```python
from build123d import *

# Parameters (mm, degrees)
SKETCH1_W                = 12.7
SKETCH1_H                = 9.525
BOSS_EXTRUDE1_DEPTH      = 9.525
BOSS_EXTRUDE1_DEPTH_BACK = 22.225
SKETCH2_W                = 28.575
SKETCH2_H                = 32.144829198
CUT_EXTRUDE1_DEPTH       = 127.92060018
CUT_EXTRUDE1_DEPTH_BACK  = 127.92060018
CHAMFER1_SIZE            = 9.525
SKETCH11_W               = 143.179068554
SKETCH11_H               = 12.488767135
CUT_EXTRUDE5_DEPTH       = 119.773497618
SKETCH5_W                = 9.85
SKETCH5_H                = 3
SKETCH5_W_2              = 60
SKETCH5_H_2              = 4
CUT_EXTRUDE3_REACH       = 156.535
SKETCH6_R                = 1.7272
SKETCH6_R_2              = 8
SKETCH7_W                = 25.4
SKETCH7_H                = 22.769743879
BOSS_EXTRUDE2_DEPTH      = 1.5875
CUT_EXTRUDE4_REACH       = 157.713
SKETCH8_R                = 3
CUT_EXTRUDE6_DEPTH       = 99.74454178
CUT_EXTRUDE6_DEPTH_BACK  = 12.7


with BuildPart() as part:
    # Sketch1 → Revolve1 (revolve)
    with BuildSketch(Plane.XY, mode=Mode.PRIVATE) as revolve1_sk:
        with Locations((-28.575, 4.7625)):
            Rectangle(SKETCH1_W, SKETCH1_H)
        with Locations((28.575, 4.7625)):
            Rectangle(SKETCH1_W, SKETCH1_H)
    revolve(revolve1_sk.sketch.rotate(Axis((-22.225, 0, 0), (1, 0, 0)), 90), axis=Axis((-22.225, 0, 0), (1, 0, 0)))

    # Sketch2 → Boss-Extrude1 (add, two sides: drawn at the far end of the back side and taken through both)
    with BuildSketch(Plane(origin=(0, 0, 0), x_dir=(1, 0, 0), z_dir=(0, 1, 0)).offset(-BOSS_EXTRUDE1_DEPTH_BACK)):
        Polygon((-57.15, 5.955170802), (-34.925, 0), (-22.225, 0), (-22.225, 25.4), (22.225, 25.4), (22.225, 0), (34.925, 0), (57.15, 5.955170802), (57.15, 101.6), (-57.15, 101.6), align=None)
        Polygon((-22.225, 28.575), (-22.225, 50.8), (-53.975, 50.8), (-53.975, 98.425), (53.975, 98.425), (53.975, 50.8), (22.225, 50.8), (22.225, 28.575), align=None, mode=Mode.SUBTRACT)
        with Locations((39.6875, 28.377585401)):
            Rectangle(SKETCH2_W, SKETCH2_H, mode=Mode.SUBTRACT)
        with Locations((-39.6875, 28.377585401)):
            Rectangle(SKETCH2_W, SKETCH2_H, mode=Mode.SUBTRACT)
    extrude(amount=BOSS_EXTRUDE1_DEPTH + BOSS_EXTRUDE1_DEPTH_BACK)

    # Sketch3 → Cut-Extrude1 (cut, two sides: drawn at the far end of the back side and taken through both)
    with BuildSketch(Plane(origin=(0, 0, -101.6), x_dir=(-1, 0, 0), z_dir=(0, 0, -1)).offset(-CUT_EXTRUDE1_DEPTH_BACK)):
        Polygon((-363.181758486, 0.544743879), (-78.360804047, 0.544743879), (-53.975, 0.544743879), (-34.925, 9.525), (34.925, 9.525), (53.975, 0.544743879), (73.137213101, 0.544743879), (357.958167541, 0.544743879), (357.958167541, 570.186652758), (-363.181758486, 570.186652758), align=None)
    extrude(amount=CUT_EXTRUDE1_DEPTH + CUT_EXTRUDE1_DEPTH_BACK, mode=Mode.SUBTRACT)

    # Chamfer1
    chamfer1_edges = [part.edges().sort_by_distance(p)[0] for p in [
        (-25.4, -6.35, -12.305170802),
        (25.4, -6.35, -12.305170802),
    ]]
    chamfer(chamfer1_edges, length=CHAMFER1_SIZE)

    # Sketch11 → Cut-Extrude5 (cut, through all)
    with BuildSketch(Plane(origin=(0, 0.544743879, 0), x_dir=(1, 0, 0), z_dir=(0, 1, 0))):
        with Locations((14.439534277, 95.355616432)):
            Rectangle(SKETCH11_W, SKETCH11_H)
    extrude(amount=CUT_EXTRUDE5_DEPTH, mode=Mode.SUBTRACT)

    # Sketch5 → Cut-Revolve1 (revolve, cut)
    with BuildSketch(Plane(origin=(0, 0, 0), x_dir=(1, 0, 0), z_dir=(0, 1, 0)), mode=Mode.PRIVATE) as cut_revolve1_sk:
        Polygon((-34.925, -3), (-34.925, 0), (-41.275, 0), (-41.275, -6.604), (-34.925, -6.604), align=None)
        with Locations((-30, -1.5)):
            Rectangle(SKETCH5_W, SKETCH5_H)
        Polygon((73.349668225, 0), (34.925, 0), (34.925, -4), (34.925, -6.604), (73.349668225, -6.604), align=None)
        with Locations((4.925, -2)):
            Rectangle(SKETCH5_W_2, SKETCH5_H_2)
    revolve(cut_revolve1_sk.sketch.rotate(Axis((116.428907087, 0, 0), (-1, 0, 0)), 180), axis=Axis((116.428907087, 0, 0), (-1, 0, 0)), mode=Mode.SUBTRACT)

    # Sketch6 → Cut-Extrude3 (cut, up to next)
    with BuildSketch(Plane.ZY.offset(57.15), mode=Mode.PRIVATE) as cut_extrude3_sk1:
        with Locations((-88.9, -9.525)):
            Circle(SKETCH6_R)
    cut_extrude3_tool1 = extrude(cut_extrude3_sk1.sketch, amount=-CUT_EXTRUDE3_REACH, mode=Mode.PRIVATE) & part.part
    # Sketch6 → Cut-Extrude3 (cut, up to next)
    with BuildSketch(Plane.ZY.offset(57.15), mode=Mode.PRIVATE) as cut_extrude3_sk2:
        with Locations((-21.830170802, -9.525)):
            Circle(SKETCH6_R)
    cut_extrude3_tool2 = extrude(cut_extrude3_sk2.sketch, amount=-CUT_EXTRUDE3_REACH, mode=Mode.PRIVATE) & part.part
    # Sketch6 → Cut-Extrude3 (cut, up to next)
    with BuildSketch(Plane.ZY.offset(57.15), mode=Mode.PRIVATE) as cut_extrude3_sk3:
        with Locations((-55.365085401, -9.525)):
            Circle(SKETCH6_R_2)
    cut_extrude3_tool3 = extrude(cut_extrude3_sk3.sketch, amount=-CUT_EXTRUDE3_REACH, mode=Mode.PRIVATE) & part.part
    cut_extrude3_1 = cut_extrude3_tool1.solids().sort_by_distance((-57.15, -9.525, -88.9))[0]
    add(cut_extrude3_1, mode=Mode.SUBTRACT)
    cut_extrude3_2 = cut_extrude3_tool2.solids().sort_by_distance((-57.15, -9.525, -21.830171))[0]
    add(cut_extrude3_2, mode=Mode.SUBTRACT)
    cut_extrude3_3 = cut_extrude3_tool3.solids().sort_by_distance((-57.15, -9.525, -55.365085))[0]
    add(cut_extrude3_3, mode=Mode.SUBTRACT)
    cut_extrude3 = cut_extrude3_1 + cut_extrude3_2 + cut_extrude3_3  # Cut-Extrude3 as one shape, for the pattern or mirror that repeats it

    # Sketch7 → Boss-Extrude2 (add)
    with BuildSketch(Plane.ZY.offset(57.15)):
        with Locations((-55.365085401, -10.840128061)):
            Rectangle(SKETCH7_W, SKETCH7_H)
    boss_extrude2 = extrude(amount=BOSS_EXTRUDE2_DEPTH)

    # Sketch8 → Cut-Extrude4 (cut, up to next)
    with BuildSketch(Plane.ZY.offset(58.7375), mode=Mode.PRIVATE) as cut_extrude4_sk1:
        with Locations((-55.365085401, -9.525)):
            Circle(SKETCH8_R)
    cut_extrude4_tool1 = extrude(cut_extrude4_sk1.sketch, amount=-CUT_EXTRUDE4_REACH, mode=Mode.PRIVATE) & part.part
    cut_extrude4 = cut_extrude4_tool1.solids().sort_by_distance((-58.7375, -9.525, -55.365085))[0]
    add(cut_extrude4, mode=Mode.SUBTRACT)

    # Mirror1: Cut-Extrude3, Boss-Extrude2, Cut-Extrude4 across plane
    add(cut_extrude3.mirror(Plane(origin=(0, 0, 0), x_dir=(0, 0, 1), z_dir=(1, 0, 0))), mode=Mode.SUBTRACT)
    add(boss_extrude2.mirror(Plane(origin=(0, 0, 0), x_dir=(0, 0, 1), z_dir=(1, 0, 0))))
    add(cut_extrude4.mirror(Plane(origin=(0, 0, 0), x_dir=(0, 0, 1), z_dir=(1, 0, 0))), mode=Mode.SUBTRACT)

    # Sketch12 → Cut-Extrude6 (cut, two sides: drawn at the far end of the back side and taken through both)
    with BuildSketch(Plane.XY.offset(-25.4).offset(-CUT_EXTRUDE6_DEPTH_BACK)):
        Polygon((-139.974688472, 150.824626166), (-22.225, 9.525), (-6.35, -9.525), (6.35, -9.525), (22.225, 9.525), (139.974688472, 150.824626166), (139.974688472, 518.686412656), (-139.974688472, 518.686412656), align=None)
    extrude(amount=CUT_EXTRUDE6_DEPTH + CUT_EXTRUDE6_DEPTH_BACK, mode=Mode.SUBTRACT)


solid = part.part
```
CAD build for the part. Positions are in the model's coordinates, mm. A direction names the side the tool comes from. Round coordinates to 2 decimals unless told otherwise and drop trailing zeros. Loops run counter-clockwise (first coordinate to the right, second up) from the corner with the lowest first, then second, coordinate; pieces in that order, holes last. Notation, with made-up numbers: (4.25, 0.25) - (41.25, 0.25) arc R15 cw to (41.25, 10.25) - close; hole circle Ø8 at (-33, 12.25). An arc over 180 degrees is marked (long way). Return JSON: item names as keys, results as strings. Group by question number.
Q1. Flat gauge pins, fed straight in: pin 1 Ø16 at (y, z) = (-13, -11.5) entering from +X; pin 2 Ø1.3 at (x, y) = (-57.5, -10) entering from +Z; pin 3 Ø10 at (x, y) = (-10.5, 0.5) entering from +Z. Where does each tip first touch, or does it go through?
Q2. Band-saw the part on D-D on z = -39.5. Give the cut face in (x, y) (3 decimals).
Q3. Band-saw the part on B-B on x = 49.5. Give the number of separate pieces and of enclosed holes in the cut face, plus the area to 3 significant figures.
Q4. Drill centre lines: line 1 along X through (y, z) = (-19.5, -39) (3 decimals); line 2 along Y through (x, z) = (-56.35, -88.9) (3 decimals); line 3 along Z through (x, y) = (18, -14) (3 decimals). Where is each one in solid material? Low to high. Write a range as [from, to].
Q5. Band-saw the part on C-C on x = -30.5. Give the cut face in (y, z) (3 decimals), plus the area to 3 significant figures.
Q6. Two-plate mould, pull along X, no slides. Class faces 4 (the face through (55.58, -9.01, -20.18)), 5 (the face through (44.583, 4.972, -47.581)), 6 (the face through (-44.317, 5.098, -7.434)), 7 (the face through (-40, -7, -44.45)): +X half, -X half, draft (parallel to the pull), parting line (faces both ways), or undercut.
Q7. Tool access for faces 1 (the face through (22.225, -7, -12)), 2 (the face through (43.724, 0.145, -6.602)), 3 (the face through (-25.075, -3, -1)): list every direction of +Z, -Z, +X, -X, +Y, -Y with a clear straight run to the whole face (end or side of a thin tool).
Q8. Band-saw the part on A-A on z = -88.9. Give the cut face in (x, y) (3 decimals), plus the area to 3 significant figures.
Solutions:
{
 "1": {"pin 1": "stops at x = 57.15", "pin 2": "stops at z = -5.87", "pin 3": "stops at z = -25.4"},
 "2": {"outline": "(-57.15, -22.225) - (-53.975, -22.225) - (-53.975, 0.545) - (-57.15, 0.545) - close; (-25.4, -22.225) - (-22.225, -22.225) - (-22.225, 9.525) - (-25.4, 9.525) - close; (22.225, -22.225) - (25.4, -22.225) - (25.4, 9.525) - (22.225, 9.525) - close; (53.975, -22.225) - (57.15, -22.225) - (57.15, 0.545) - (53.975, 0.545) - close"},
 "3": {"separate pieces": "3", "enclosed holes": "0", "area": "391 mm^2"},
 "4": {"line 1": "x = [-57.15, -53.975], [-25.4, -22.225], [22.225, 25.4], [53.975, 57.15]", "line 2": "y = [-22.225, -11.252], [-7.798, 0.545]", "line 3": "z = [-101.6, -98.425], [-28.575, -25.4]"},
 "5": {"outline": "(-22.225, -101.6) - (0.545, -101.6) - (0.545, -98.425) - (-22.225, -98.425) - close; (-22.225, -50.8) - (-16.095, -50.8) arc R8 cw to (-2.955, -50.8) - (9.525, -50.8) - (9.525, -44.45) - (-22.225, -44.45) - close; (-22.225, -16.73) - (9.525, -16.73) - (9.525, 0) arc R9.525 ccw to (-9.525, 0) - (-22.225, 0) - close; hole circle Ø6 at (0, 0)", "area": "888 mm^2"},
 "6": {"face 4": "draft", "face 5": "+X half", "face 6": "-X half", "face 7": "undercut"},
 "7": {"face 1": "+Z, +Y, -Y", "face 2": "+Z, +X", "face 3": "+X"},
 "8": {"outline": "(-57.15, -22.225) - (-53.975, -22.225) - (-53.975, -11.252) - (-57.15, -11.252) - close; (-57.15, -7.798) - (-53.975, -7.798) - (-53.975, 0.545) - (-57.15, 0.545) - close; (53.975, -22.225) - (57.15, -22.225) - (57.15, -11.252) - (53.975, -11.252) - close; (53.975, -7.798) - (57.15, -7.798) - (57.15, 0.545) - (53.975, 0.545) - close", "area": "123 mm^2"}
}
